Read the model definition and answer for the solid it produces. Units are mm, in the model's axes. A direction names the side the tool comes from. Give positions to 0.01 mm unless a question says otherwise; leave off trailing zeros. Order: outer loops, then holes, each group sorted by start corner. A loop starts at its lowest first (then second) coordinate and runs counter-clockwise, first axis right, second up. Notation, with made-up numbers: (48.5, 46) - (72.5, 46) arc R22 ccw to (72.5, 76) - close; hole circle Ø11 at (26.5, 29.25). An arc over 180 degrees is marked (long way). Use a Markdown table: item, result. Add a question column.
1. Flat-ended cylindrical pins translate along their axes: P1, Ø3, axis at x = 8, y = -1.5, coming from the -Z side; P2, Ø2.5, axis at x = -14, y = -0.5, coming from the +Z side; P3, Ø2.5, axis at y = 1, z = 16.5, coming from the -X side. Find the tip coordinate at first contact, or state that the pin passes through.
2. Consider L1, parallel to Z at x = 0, y = 1.25; L2, parallel to X at y = 2, z = -22; L3, parallel to Z at x = -14, y = -1.25. Determine where each line is inside the solid, lowest interval first.
3. A cutting plane is placed at D-D on x = -27. Determine the outline of the cut face in (y, z), and give its area (3 significant figures).
4. For a pull along X with two mould halves and no side action, classify faces 3 (the flat face through (5, 0, 18)), 4 (the cylindrical face through (-40, 0, 0)), 5 (the cylindrical face through (28.022, -0.035, -28.544)) as released by +X, released by -X, zero draft, split by the parting line, or undercut.
5. Which of the six approach directions +Z, -Z, +X, -X, +Y, -Y give full straight-line access (tool end or side, diameter ignored) to faces 1 (the cylindrical face through (-28.544, -0.035, -28.022)), 2 (the flat face through (-18, 0, 5))?
6. A cutting plane is placed at C-C on z = 15. Determine the outline of the cut face in (x, y), and give its area (3 significant figures).
7. A cutting plane is placed at B-B on y = 0.05. Determine the outline of the cut face in (x, z), and give its area (3 significant figures).
8. A cutting plane is placed at A-A on x = 0. Determine the outline of the cut face in (y, z), and give its area (3 significant figures).
```python
from build123d import *

# Parameters (mm, degrees)
F0_R     = 2.5
F1_DEPTH = 2.5


with BuildPart() as f1:
    # F0 (on Front) → F1 (new body, symmetric)
    with BuildSketch(Plane.XZ):
        with BuildLine():
            ThreePointArc((39.68627, -5), (39.92149, -2.504917), (40, 0))
            ThreePointArc((40, 0), (39.92149, 2.504917), (39.68627, 5))
            ThreePointArc((39.68627, 5), (28.284271, 28.284271), (5, 39.68627))
            ThreePointArc((5, 39.68627), (0, 40), (-5, 39.68627))
            ThreePointArc((-5, 39.68627), (-28.284271, 28.284271), (-39.68627, 5))
            ThreePointArc((-39.68627, 5), (-40, 0), (-39.68627, -5))
            ThreePointArc((-39.68627, -5), (-28.284271, -28.284271), (-5, -39.68627))
            ThreePointArc((-5, -39.68627), (0, -40), (5, -39.68627))
            ThreePointArc((5, -39.68627), (28.284271, -28.284271), (39.68627, -5))
        make_face()
        with BuildLine():
            Line((-5.59017, -5), (-5, -5))
            Line((-5, -5), (-5, -30.594117))
            ThreePointArc((-5, -30.594117), (-21.92031, -21.92031), (-30.594117, -5))
            Line((-30.594117, -5), (-5.59017, -5))
        make_face(mode=Mode.SUBTRACT)
        with BuildLine():
            Line((5, -30.594117), (5, -5.59017))
            ThreePointArc((5, -5.59017), (5.303301, -5.303301), (5.59017, -5))
            Line((5.59017, -5), (30.594117, -5))
            ThreePointArc((30.594117, -5), (21.92031, -21.92031), (5, -30.594117))
        make_face(mode=Mode.SUBTRACT)
        with BuildLine():
            Line((-5, 30.594117), (-5, 5))
            Line((-5, 5), (-30.594117, 5))
            ThreePointArc((-30.594117, 5), (-21.92031, 21.92031), (-5, 30.594117))
        make_face(mode=Mode.SUBTRACT)
        Circle(F0_R, mode=Mode.SUBTRACT)
        with BuildLine():
            ThreePointArc((5, 30.594117), (21.92031, 21.92031), (30.594117, 5))
            Line((30.594117, 5), (5.59017, 5))
            ThreePointArc((5.59017, 5), (5.303301, 5.303301), (5, 5.59017))
            Line((5, 5.59017), (5, 30.594117))
        make_face(mode=Mode.SUBTRACT)
    extrude(amount=F1_DEPTH, both=True)


solid = f1.part
```
Output values:
| question | item | result |
|---|---|---|
| 1 | P1 | z = -39.47 |
| 1 | P2 | z = 37.91 |
| 1 | P3 | x = -36.98 |
| 2 | L1 | -40 to -2.5, 2.5 to 40 |
| 2 | L2 | -33.41 to -21.84, -5 to 5, 21.84 to 33.41 |
| 2 | L3 | -37.47 to -27.66, -5 to 5, 27.66 to 37.47 |
| 3 | outline | (-2.5, -29.51) - (2.5, -29.51) - (2.5, -15.23) - (-2.5, -15.23) - close; (-2.5, -5) - (2.5, -5) - (2.5, 5) - (-2.5, 5) - close; (-2.5, 15.23) - (2.5, 15.23) - (2.5, 29.51) - (-2.5, 29.51) - close |
| 3 | area | 193 mm² |
| 4 | face 3 | undercut |
| 4 | face 4 | released by -X |
| 4 | face 5 | released by +X |
| 5 | face 1 | -Z, -X, +Y, -Y |
| 5 | face 2 | +Y, -Y |
| 6 | outline | (-37.08, -2.5) - (-27.13, -2.5) - (-27.13, 2.5) - (-37.08, 2.5) - close; (-5, -2.5) - (5, -2.5) - (5, 2.5) - (-5, 2.5) - close; (27.13, -2.5) - (37.08, -2.5) - (37.08, 2.5) - (27.13, 2.5) - close |
| 6 | area | 150 mm² |
| 7 | outline | (-39.69, -5) arc R40 ccw to (-5, -39.69) arc R40 ccw to (5, -39.69) arc R40 ccw to (39.69, -5) arc R40 ccw to (40, 0) arc R40 ccw to (39.69, 5) arc R40 ccw to (5, 39.69) arc R40 ccw to (-5, 39.69) arc R40 ccw to (-39.69, 5) arc R40 ccw to start; hole (-30.59, -5) arc R31 ccw to (-5, -30.59) - (-5, -5) - close; hole (-30.59, 5) - (-5, 5) - (-5, 30.59) arc R31 ccw to start; hole circle Ø5 at (0, 0); hole (5, -30.59) arc R31 ccw to (30.59, -5) - (5.59, -5) arc R7.5 cw to (5, -5.59) - close; hole (5, 5.59) arc R7.5 cw to (5.59, 5) - (30.59, 5) arc R31 ccw to (5, 30.59) - close |
| 7 | area | 3,120 mm² |
| 8 | outline | (-2.5, -40) - (2.5, -40) - (2.5, -2.5) - (-2.5, -2.5) - close; (-2.5, 2.5) - (2.5, 2.5) - (2.5, 40) - (-2.5, 40) - close |
| 8 | area | 375 mm² |
